Geometry check sheet. Reference: the model listing, model coordinates, mm. A direction names the side the tool comes from. Give positions to 0.01 mm unless a question says otherwise; leave off trailing zeros. Loops run counter-clockwise (first coordinate to the right, second up) from the corner with the lowest first, then second, coordinate; pieces in that order, holes last. Notation, with made-up numbers: (86.5, 13.25) -> (96.5, 13.25) arc R24 ccw to (96.5, 34.25) -> close; hole circle Ø5 at (58, 23). An arc over 180 degrees is marked (long way). One line per item, written item: value. Start each with the question number.
(1) Tool access check on faces 1 (the face through (-2.839, 16.806, -8.493)), 2 (the face through (-2.839, 16.806, 8.493)), 3 (the face through (-5, 20, -9)), 4 (the face through (-5, 20, 9)), 5 (the face through (-10.81, 1.01, 6.66)). Record the directions out of +Z, -Z, +X, -X, +Y, -Y that give a thin tool (end or side, any length) a straight path to the whole face; none if there is none.
(2) Sectioned sample at A-A, the plane z = 25.5. Record the cut outline in (x, y).
(3) Sectioned sample at C-C, the plane y = 8. Record the cut outline in (x, z).
(4) Draft check along X on faces 6 (the face through (6.121, 1.014, 22.753)), 7 (the face through (-10.84, 1.01, -32.81)), 8 (the face through (-5.15, 17.07, 0.08)). Enter one of: pulls with the +X half, pulls with the -X half, needs draft (parallel to the pull), parting line crosses it, or undercut.
(5) Sectioned sample at B-B, the plane x = -4.5. State how many separate pieces and enclosed holes the cut face has, then the cut area to 3 significant figures.
(6) Scan lines: line 1 along Z through (x, y) = (3.75, 6.5); line 2 along X through (y, z) = (1.55, 25.5); line 3 along Y through (x, z) = (-0.5, 27). Record each from-to range of solid material in increasing order. Write a range as from..to.
(7) Gauge pin test, flat ends, axial feed: pin 1 Ø7.5 at (x, y) = (-6.5, 16.5) entering from -Z; pin 2 Ø8 at (x, y) = (-1, 16.5) entering from +Z; pin 3 Ø2 at (y, z) = (7, 7) entering from -X; pin 4 Ø5 at (x, z) = (6, -25.5) entering from -Y. Record the tip position at first contact, or that the pin passes through.
(8) Sectioned sample at D-D, the plane y = 20. Record the cut outline in (x, z), then the cut area to 3 significant figures.
from build123d import *

# Parameters (mm, degrees)
EXTRUDE_START       = 33.5
SKETCH_3_W          = 23
SKETCH_3_H          = 2
EXTRUDE_1_DEPTH     = 67
EXTRUDE_START_2     = 8
SKETCH_4_R          = 3
EXTRUDE_2_DEPTH     = 2
EXTRUDE_START_3     = -6
SKETCH_5_R          = 3
EXTRUDE_3_DEPTH     = 2
SKETCH_6_R          = 3.6
EXTRUDE_4_DEPTH     = 1
EXTRUDE_START_4     = 16
SKETCH_7_R          = 3
EXTRUDE_5_DEPTH     = 16
SKETCH_8_W          = 12
SKETCH_8_H          = 12.516134774
CUT_EXTRUDE_1_DEPTH = 23
SKETCH_9_R          = 2.75
CUT_EXTRUDE_2_DEPTH = 46.094345544
FILLET_3_R          = 2.3


with BuildPart() as part:
    # 草图3 → 凸台-拉伸1 (new body)
    with BuildSketch(Plane.XY.offset(EXTRUDE_START)):
        with Locations((0, 1)):
            Rectangle(SKETCH_3_W, SKETCH_3_H)
    extrude(amount=-EXTRUDE_1_DEPTH)

    # 草图4 → 凸台-拉伸2 (add)
    with BuildSketch(Plane.XY.offset(EXTRUDE_START_2)):
        with BuildLine():
            Line((-8.1, 11.751363749), (-8.1, 0))
            Line((-8.1, 0), (11.5, 0))
            Line((11.5, 0), (11.5, 2))
            Line((11.5, 2), (3.973803242, 23.032269549))
            ThreePointArc((3.973803242, 23.032269549), (-10.644363142, 26.576230043), (-8.1, 11.751363749))
        make_face()
        with Locations((-4.5, 20)):
            Circle(SKETCH_4_R, mode=Mode.SUBTRACT)
    extrude(amount=-EXTRUDE_2_DEPTH)

    # 草图5 → 凸台-拉伸3 (add)
    with BuildSketch(Plane.XY.offset(EXTRUDE_START_3)):
        with BuildLine():
            Line((-8.1, 11.751363749), (-8.1, 0))
            Line((-8.1, 0), (11.5, 0))
            Line((11.5, 0), (11.5, 2))
            Line((11.5, 2), (3.973803242, 23.032269549))
            ThreePointArc((3.973803242, 23.032269549), (-10.644363142, 26.576230043), (-8.1, 11.751363749))
        make_face()
        with Locations((-4.5, 20)):
            Circle(SKETCH_5_R, mode=Mode.SUBTRACT)
    extrude(amount=-EXTRUDE_3_DEPTH)

    # 草图6 → 凸台-拉伸4 (add)
    with BuildSketch(Plane.XY.offset(8)):
        with Locations((-4.5, 20)):
            Circle(SKETCH_6_R)
    extrude_4 = extrude(amount=EXTRUDE_4_DEPTH)

    # 镜向2: 凸台-拉伸4 across plane
    add(extrude_4.mirror(Plane.XY))

    # 草图7 → 凸台-拉伸5 (add)
    with BuildSketch(Plane.XY.offset(-8).offset(EXTRUDE_START_4)):
        with Locations((-4.5, 20)):
            Circle(SKETCH_7_R)
    extrude(amount=-EXTRUDE_5_DEPTH)

    # 草图8 → 切除-拉伸1 (cut)
    with BuildSketch(Plane(origin=(11.5, 0, 0), x_dir=(0, 0, -1), z_dir=(1, 0, 0))):
        with Locations((0, 6.258067387)):
            Rectangle(SKETCH_8_W, SKETCH_8_H)
    extrude(amount=-CUT_EXTRUDE_1_DEPTH, mode=Mode.SUBTRACT)

    # 草图9 → 切除-拉伸2 (cut, through all)
    with BuildSketch(Plane(origin=(0, 2, 0), x_dir=(1, 0, 0), z_dir=(0, 1, 0))):
        with Locations(Location((-6, 25.5, 0), (0, 0, 270))):
            Circle(SKETCH_9_R)
        with Locations(Location((6, 25.5, 0), (0, 0, 90))):
            Circle(SKETCH_9_R)
        with Locations(Location((6, -25.5, 0), (0, 0, 270))):
            Circle(SKETCH_9_R)
        with Locations(Location((-6, -25.5, 0), (0, 0, 90))):
            Circle(SKETCH_9_R)
    extrude(amount=-CUT_EXTRUDE_2_DEPTH, mode=Mode.SUBTRACT)

    # 圆角3
    fillet_3_edges = [part.edges().sort_by_distance(p)[0] for p in [
        (-11.5, 1, -33.5),
        (-11.5, 1, 33.5),
        (11.5, 1, 33.5),
        (11.5, 1, -33.5),
        (-11.5, 1, -6),
        (-11.5, 1, 6),
    ]]
    fillet(fillet_3_edges, radius=FILLET_3_R)


solid = part.part
Calculated:
1. face 1: -Z
1. face 2: +Z
1. face 3: -Z, +X, -X, +Y
1. face 4: +Z, +X, -X, +Y
1. face 5: -X, -Y
2. outline: (-11.5, 0) -> (-8.75, 0) -> (-8.75, 2) -> (-11.5, 2) -> close; (-3.25, 0) -> (3.25, 0) -> (3.25, 2) -> (-3.25, 2) -> close; (8.75, 0) -> (11.5, 0) -> (11.5, 2) -> (8.75, 2) -> close
3. outline: (-8.1, -8) -> (9.35, -8) -> (9.35, -6) -> (-8.1, -6) -> close; (-8.1, 6) -> (9.35, 6) -> (9.35, 8) -> (-8.1, 8) -> close
4. face 6: undercut
4. face 7: pulls with the -X half
4. face 8: parting line crosses it
5. separate pieces: 3
5. enclosed holes: 0
5. area: 286 mm2
6. line 1: z = -8..-6, 6..8
6. line 2: x = -11.5..-8.75, -3.25..3.25, 8.75..11.5
6. line 3: y = 0..2
7. pin 1: stops at z = -9
7. pin 2: stops at z = 9
7. pin 3: stops at x = -8.1
7. pin 4: passes through
8. outline: (-13.5, -8) -> (-8.1, -8) -> (-8.1, -9) -> (-0.9, -9) -> (-0.9, -8) -> (5.06, -8) -> (5.06, -6) -> (-1.5, -6) -> (-1.5, 6) -> (5.06, 6) -> (5.06, 8) -> (-0.9, 8) -> (-0.9, 9) -> (-8.1, 9) -> (-8.1, 8) -> (-13.5, 8) -> (-13.5, 6) -> (-7.5, 6) -> (-7.5, -6) -> (-13.5, -6) -> close
8. area: 161 mm2
